Work out the finished part from the listing and answer in its coordinate system (mm). A direction names the side the tool comes from. Round coordinates to 2 decimals unless told otherwise and drop trailing zeros. Loops run counter-clockwise (first coordinate to the right, second up) from the corner with the lowest first, then second, coordinate; pieces in that order, holes last. Notation, with made-up numbers: (-26.5, 22.25) -> (-4.5, 22.25) arc R25 cw to (-4.5, 40.25) -> close; hole circle Ø9 at (47, 16). An arc over 180 degrees is marked (long way). Use one line per item in the form item = value.
```python
from build123d import *

# Parameters (mm, degrees)
F1_DEPTH = 76.2
F2_DEPTH = 25.4
F4_DEPTH = 127


with BuildPart() as f1:
    # F0 (on Front) → F1 (new body)
    with BuildSketch(Plane.XZ):
        Polygon((0, 16.379364), (0, 0), (76.2, 0), (76.2, 25.4), (63.5, 25.4), (63.5, 127), (50.8, 127), (31.600004, 510.643689), (0, 29.079364), (12.7, 29.079364), (12.7, 16.379364), align=None)
    extrude(amount=F1_DEPTH)

    # F0 (on Front) + F1_face (on face) → F2 (join)
    with BuildSketch(Plane.XZ):
        Polygon((0, 16.379364), (0, 0), (76.2, 0), (76.2, 25.4), (63.5, 25.4), (63.5, 127), (50.8, 127), (31.600004, 510.643689), (0, 29.079364), (12.7, 29.079364), (12.7, 16.379364), align=None)
    with BuildSketch(Plane(origin=(32.20504, -76.2, 161.502692), x_dir=(1, 0, 0), z_dir=(0, -1, 0))):
        Polygon((-32.20504, -132.423328), (-19.50504, -132.423328), (-19.50504, -145.123328), (-32.20504, -145.123328), (-32.20504, -161.502692), (43.99496, -161.502692), (43.99496, -136.102692), (31.29496, -136.102692), (31.29496, -34.502692), (18.59496, -34.502692), (-0.605036, 349.140998), align=None)
    extrude(amount=F2_DEPTH)

    # F3 (on Right) → F4 (cut, symmetric)
    with BuildSketch(Plane.YZ):
        Polygon((-53.018704, 510.999203), (36.268413, 0), (28.625131, 603.81484), (-150.899715, 678.91259), (-142.305821, 0), align=None)
    extrude(amount=F4_DEPTH, both=True, mode=Mode.SUBTRACT)


solid = f1.part
```
(1) Find section D-D, the plane y = -39.5. Write down the section's boundary in (x, z), then the cut area to 3 significant figures.
Completed:
outline = (0, 0) -> (76.2, 0) -> (76.2, 25.4) -> (63.5, 25.4) -> (63.5, 127) -> (50.8, 127) -> (35.45, 433.63) -> (26.55, 433.63) -> (0, 29.08) -> (12.7, 29.08) -> (12.7, 16.38) -> (0, 16.38) -> close
area = 16,100 mm2
(2) Find section C-C, the plane z = 358.5. Write down the section's boundary in (x, y), then the cut area to 3 significant figures.
Completed:
outline = (21.62, -79.66) -> (39.21, -79.66) -> (39.21, -26.37) -> (21.62, -26.37) -> close
area = 938 mm2
(3) For faces 4 (the flat face through (12.7, -50, 23)), 5 (the flat face through (70, -50, 25.4)), 6 (the flat face through (38, -101.6, 92)), determine the directions among +Z, -Z, +X, -X, +Y, -Y from which every point of the face is accessible in a straight line to the end or side of a thin tool.
Completed:
face_4 = -X, +Y, -Y
face_5 = +Z, +X, +Y, -Y
face_6 = +Z, -Z, +X, -X, -Y
(4) Given P1, Ø8, axis at y = -71.5, z = 86, coming from the -X side; P2, Ø6.5, axis at y = -50.5, z = 25, coming from the -X side; P3, Ø14, axis at x = 70, y = -68.5, coming from the +Z side, each flat-ended and moving along its own axis, determine where each tip first touches the part or whether it passes through.
Completed:
P1 = 3.47
P2 = 12.7
P3 = 127
(5) Consider L1, parallel to Z at x = 65.5, y = -60; L2, parallel to Z at x = 60.5, y = -59.5; L3, parallel to X at y = -10.5, z = 173.5. Determine where each line is inside the solid, lowest interval first.
Completed:
L1 = 0 to 25.4
L2 = 0 to 127
L3 = 9.48 to 48.47
(6) Find section B-B, the plane y = -68.5. Write down the section's boundary in (x, z).
Completed:
outline = (0, 0) -> (76.2, 0) -> (76.2, 25.4) -> (63.5, 25.4) -> (63.5, 127) -> (50.8, 127) -> (36.02, 422.4) -> (25.81, 422.4) -> (0, 29.08) -> (12.7, 29.08) -> (12.7, 16.38) -> (0, 16.38) -> close
(7) Find section A-A, the plane x = 5. Write down the section's boundary in (y, z).
Completed:
outline = (-101.6, 0) -> (0, 0) -> (0, 16.38) -> (-101.6, 16.38) -> close; (-101.6, 29.08) -> (0, 29.08) -> (0, 105.28) -> (-101.6, 105.28) -> close
(8) For a pull along Z with two mould halves and no side action, classify faces 1 (the flat face through (0, -50, 8)), 2 (the flat face through (6, -50, 16.379)), 3 (the flat face through (38, -50, 0)) as +Z half, -Z half, draft (parallel to the pull), parting line (faces both ways), or undercut.
Completed:
face_1 = draft
face_2 = undercut
face_3 = -Z half
